Could you check a few things on this drawing? It's one solid part, dimensions in mm from its lowest x, y, z. A direction names the side the tool comes from. Round coordinates to 2 decimals unless told otherwise and drop trailing zeros. Write each loop counter-clockwise with the first axis right and the second up, starting at its lowest first coordinate (ties: lowest second). Pieces come first, ordered by that corner, then holes. Notation, with made-up numbers: (69.5, 73) - (114.5, 73) arc R26 ccw to (114.5, 92) - close; hole circle Ø6 at (-13, 39). An arc over 180 degrees is marked (long way). Write item = value, one per line. Start each with the question number.
Item 1: If I drill on line 1 along X through (y, z) = (1, 113); line 2 along X through (y, z) = (28.5, 79); line 3 along Z through (x, y) = (17, 19), over which ranges is the centre line in solid material (lowest first)? Write a range as [from, to].
Item 2: If we section it at C-C (z = 73): Please give me the cut outline in (x, y), and give its area (3 significant figures).
Item 3: If we section it at B-B (x = 19): Please give me the cut outline in (y, z), and give its area (3 significant figures).
Item 4: Thinking about a two-plate mould opening in Z: for the marked faces 1, 2, 3 and 4, which applies, pulls with the +Z half, pulls with the -Z half, needs draft (parallel to the pull), parting line crosses it, or undercut?
Item 5: If we section it at A-A (z = 4): Please give me the cut outline in (x, y), and give its area (3 significant figures).
Item 6: If we section it at D-D (y = 12.5): Please give me the cut outline in (x, z), and give its area (3 significant figures).
Item 7: For P1, Ø4, axis at x = 15, z = 3, coming from the -Y side; P2, Ø4, axis at x = 23.5, y = 12.5, coming from the -Z side; P3, Ø2.5, axis at x = 4, z = 113, coming from the -Y side; P4, Ø4, axis at x = 18, z = 42.5, coming from the -Y side, each with a flat end and sliding along its axis, tell me the tip position at first contact or that it passes through.
Item 8: Which directions (+Z, -Z, +X, -X, +Y, -Y) give clear straight access to the entire face, cutting with the end or side of a thin tool? Please do the marked faces 5 and 6.
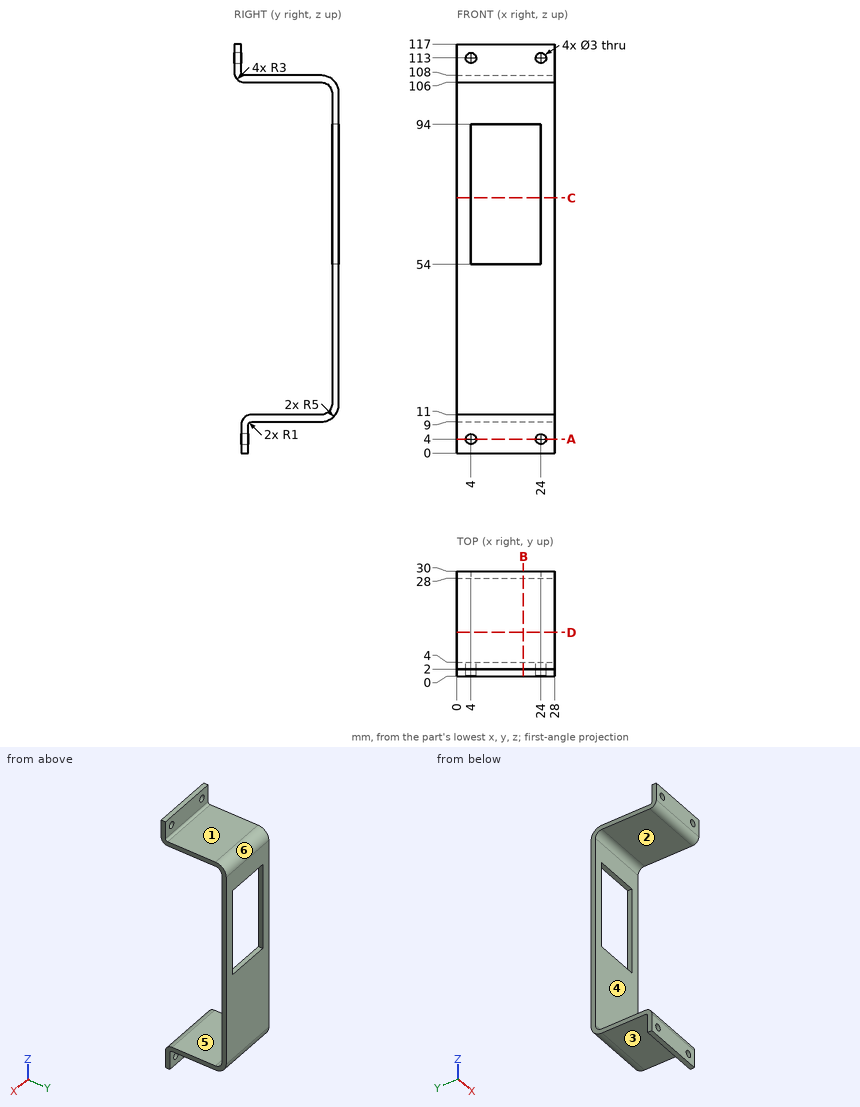
Reply:
q1.line_1 = [0, 2.5], [5.5, 22.5], [25.5, 28]
q1.line_2 = [0, 4], [24, 28]
q1.line_3 = [9, 11], [106, 108]
q2.outline = (0, 28) - (4, 28) - (4, 30) - (0, 30) - close; (24, 28) - (28, 28) - (28, 30) - (24, 30) - close
q2.area = 16.0 mm2
q3.outline = (0, 109) arc R3 ccw to (3, 106) - (25, 106) arc R3 cw to (28, 103) - (28, 94) - (30, 94) - (30, 103) arc R5 ccw to (25, 108) - (3, 108) arc R1 cw to (2, 109) - (2, 117) - (0, 117) - close; (2, 0) - (4, 0) - (4, 8) arc R1 cw to (5, 9) - (25, 9) arc R5 ccw to (30, 14) - (30, 54) - (28, 54) - (28, 14) arc R3 cw to (25, 11) - (5, 11) arc R3 ccw to (2, 8) - close
q3.area = 252 mm2
q4.face_1 = pulls with the +Z half
q4.face_2 = undercut
q4.face_3 = pulls with the -Z half
q4.face_4 = undercut
q5.outline = (0, 2) - (2.5, 2) - (2.5, 4) - (0, 4) - close; (5.5, 2) - (22.5, 2) - (22.5, 4) - (5.5, 4) - close; (25.5, 2) - (28, 2) - (28, 4) - (25.5, 4) - close
q5.area = 44.0 mm2
q6.outline = (0, 9) - (28, 9) - (28, 11) - (0, 11) - close; (0, 106) - (28, 106) - (28, 108) - (0, 108) - close
q6.area = 112 mm2
q7.P1 = 2
q7.P2 = 9
q7.P3 = through
q7.P4 = 28
q8.face_5 = +X, -X, -Y
q8.face_6 = +Z, +X, -X, +Y
